Verification items for the finished model (mm, model axes). A direction names the side the tool comes from. Coordinates: 2 decimals unless noted, no trailing zeros. Write each loop counter-clockwise with the first axis right and the second up, starting at its lowest first coordinate (ties: lowest second). Pieces come first, ordered by that corner, then holes. Notation, with made-up numbers: (39, 11.5) -> (43, 11.5) arc R8 cw to (43, 26.5) -> close; hole circle Ø2 at (-8.75, 15.5). An arc over 180 degrees is marked (long way). Answer in a Markdown table with one row per item.
```python
from build123d import *

# Parameters (mm, degrees)
CYLINDER003_R     = 5.5
CYLINDER003_DEPTH = 5
CYLINDER002_R     = 4.5
CYLINDER002_DEPTH = 6.6


with BuildPart() as centre002:
    # Cylinder003 → Cylinder003 (new body)
    with BuildSketch(Plane.XY.offset(-2.5)):
        Circle(CYLINDER003_R)
    extrude(amount=CYLINDER003_DEPTH)


with BuildPart() as worm_driven_gear:
    # Cylinder002 → Cylinder002 (new body)
    with BuildSketch(Plane.XY.offset(-9)):
        Circle(CYLINDER002_R)
    extrude(amount=CYLINDER002_DEPTH)

    # Fusion: union centre002
    add(centre002.part)


with BuildPart() as worm_driven_gear_1:
    # Fusion placement: moved
    add(worm_driven_gear.part.moved(Location((0, 0, 25))))


solid = worm_driven_gear_1.part
```
1. Section check D-D, the plane z = 24. Record the boundary of the cut face in (x, y).
Geometry says:
| item | result |
|---|---|
| outline | circle Ø11 at (0, 0) |
2. Depth check by flat-ended pin: P1, Ø3, axis at x = 0, z = 20.5, coming from the -Y side; P2, Ø6, axis at x = -0.5, z = 19, coming from the +Y side. Enter the tip coordinate at first touch or a pass-through.
Geometry says:
| item | result |
|---|---|
| P1 | y = -4.5 |
| P2 | y = 4.5 |
3. Section check C-C, the plane z = 20. Record the boundary of the cut face in (x, y).
Geometry says:
| item | result |
|---|---|
| outline | circle Ø9 at (0, 0) |
4. Section check A-A, the plane x = 0. Record the boundary of the cut face in (y, z).
Geometry says:
| item | result |
|---|---|
| outline | (-5.5, 22.5) -> (-4.5, 22.5) -> (-4.5, 16) -> (4.5, 16) -> (4.5, 22.5) -> (5.5, 22.5) -> (5.5, 27.5) -> (-5.5, 27.5) -> close |
5. Tool access check on faces 1 (the flat face through (0, 0, 27.5)), 2 (the cylindrical face through (-0.59, 4.46, 19.2)). Record the directions out of +Z, -Z, +X, -X, +Y, -Y that give a thin tool (end or side, any length) a straight path to the whole face; none if there is none.
Geometry says:
| item | result |
|---|---|
| face 1 | +Z, +X, -X, +Y, -Y |
| face 2 | -Z |
6. Thickness scan on line 1 (Z direction, x = -5, y = -2); line 2 (Y direction, x = 1, z = 24.25); line 3 (X direction, y = 3.75, z = 19.5). Record the ranges inside material, lowest first. Write a range as from..to.
Geometry says:
| item | result |
|---|---|
| line 1 | 22.5..27.5 |
| line 2 | -5.41..5.41 |
| line 3 | -2.49..2.49 |
